```python
from build123d import *

# Parameters (mm, degrees)
SKETCH1_W           = 279.4
SKETCH1_H           = 279.4
SKETCH1_R           = 11.1125
BOSS_EXTRUDE1_DEPTH = 3.175
SKETCH2_R           = 3.175
SKETCH2_R_2         = 4.7625
CUT_EXTRUDE1_DEPTH  = 198.591145108


with BuildPart() as part:
    # Sketch1 → Boss-Extrude1 (new body)
    with BuildSketch(Plane(origin=(0, 0, 0), x_dir=(1, 0, 0), z_dir=(0, 1, 0))):
        Rectangle(SKETCH1_W, SKETCH1_H)
        with Locations(Location((0, 0, 0), (0, 0, 270))):
            Circle(SKETCH1_R, mode=Mode.SUBTRACT)
    extrude(amount=BOSS_EXTRUDE1_DEPTH)

    # Sketch2 → Cut-Extrude1 (cut, through all)
    with BuildSketch(Plane(origin=(0, 3.175, 0), x_dir=(1, 0, 0), z_dir=(0, 1, 0))):
        with Locations(Location((0, 120.65, 0), (0, 0, 270))):
            Circle(SKETCH2_R)
        with Locations(Location((120.65, 0, 0), (0, 0, 270))):
            Circle(SKETCH2_R)
        with Locations(Location((0, -120.65, 0), (0, 0, 270))):
            Circle(SKETCH2_R)
        with Locations(Location((-120.65, 0, 0), (0, 0, 270))):
            Circle(SKETCH2_R)
        with Locations(Location((-120.65, 120.65, 0), (0, 0, 270))):
            Circle(SKETCH2_R_2)
        with Locations(Location((120.65, 120.65, 0), (0, 0, 90))):
            Circle(SKETCH2_R_2)
        with Locations(Location((-120.65, -120.65, 0), (0, 0, 90))):
            Circle(SKETCH2_R_2)
        with Locations(Location((120.65, -120.65, 0), (0, 0, 270))):
            Circle(SKETCH2_R_2)
    extrude(amount=-CUT_EXTRUDE1_DEPTH, mode=Mode.SUBTRACT)


solid = part.part
```
The listing builds one solid part. Answer for the finished solid, in the listing's coordinates (mm). Coordinates: 2 decimals unless noted, no trailing zeros. Write each loop counter-clockwise with the first axis right and the second up, starting at its lowest first coordinate (ties: lowest second). Pieces come first, ordered by that corner, then holes.
Q1. Given P1, Ø5, axis at x = 0, z = 120.65, coming from the -Y side, flat-ended and moving along its own axis, determine where the tip first touches the part or whether it passes through.
Returned:
P1: passes through
Q2. Find the intervals of material crossed by line 1 along X through (y, z) = (1.3, 120.65) (1 decimal); line 2 along X through (y, z) = (2.85, -120); line 3 along Z through (x, y) = (118.5, 2.5), in increasing order.
Returned:
line 1: x = -139.7 to -125.4, -115.9 to -3.2, 3.2 to 115.9, 125.4 to 139.7
line 2: x = -139.7 to -125.37, -115.93 to -3.11, 3.11 to 115.93, 125.37 to 139.7
line 3: z = -139.7 to -124.9, -116.4 to -2.34, 2.34 to 116.4, 124.9 to 139.7
Q3. Section A-A, the plane x = 0 is taken. Write down the section's boundary in (y, z) (1 decimal).
Returned:
outline: (0, -139.7) - (3.2, -139.7) - (3.2, -123.8) - (0, -123.8) - close; (0, -117.5) - (3.2, -117.5) - (3.2, -11.1) - (0, -11.1) - close; (0, 11.1) - (3.2, 11.1) - (3.2, 117.5) - (0, 117.5) - close; (0, 123.8) - (3.2, 123.8) - (3.2, 139.7) - (0, 139.7) - close
Q4. The mould has two halves that part along Z. Classify faces 1 (the cylindrical face through (116, 1.61, 119.62)), 2 (the flat face through (-33, 3.175, -2)): released by +Z, released by -Z, zero draft, split by the parting line, or undercut.
Returned:
face 1: undercut
face 2: zero draft
Q5. Section B-B, the plane z = 120.65 is taken. Write down the section's boundary in (x, y) (1 decimal), then the cut area to 3 significant figures.
Returned:
outline: (-139.7, 0) - (-125.4, 0) - (-125.4, 3.2) - (-139.7, 3.2) - close; (-115.9, 0) - (-3.2, 0) - (-3.2, 3.2) - (-115.9, 3.2) - close; (3.2, 0) - (115.9, 0) - (115.9, 3.2) - (3.2, 3.2) - close; (125.4, 0) - (139.7, 0) - (139.7, 3.2) - (125.4, 3.2) - close
area: 806 mm2
